Source: three-view drawing plus pictorial views. Frame: mm from the lowest corner of the part. Give positions to 0.01 mm unless a question says otherwise; leave off trailing zeros. Order: outer loops, then holes, each group sorted by start corner. A loop starts at its lowest first (then second) coordinate and runs counter-clockwise, first axis right, second up. Notation, with made-up numbers: (-5, 71) -> (10, 71) arc R15 ccw to (10, 80) -> close; hole circle Ø5 at (68.5, 26). An arc over 180 degrees is marked (long way). Answer in a Markdown table with one row per item. Add a question column.
Q1. Cut plane A-A on z = 7.53. Return the cut outline in (x, y), and give its area (3 significant figures).
Q2. Line query: line 1 along X through (y, z) = (20.5, 7). Output: solid intervals per line, ascending. Write a range as from..to.
Q3. Cut plane C-C on z = 10. Return the cut outline in (x, y).
Q4. Contact query for a flat-ended pin moving along its axis: P1, Ø6, axis at y = 8.5, z = 8, coming from the +X side. Output: stop coordinate, or through.
Q5. Cut plane B-B on y = 21. Return the cut outline in (x, z), and give its area (3 significant figures).
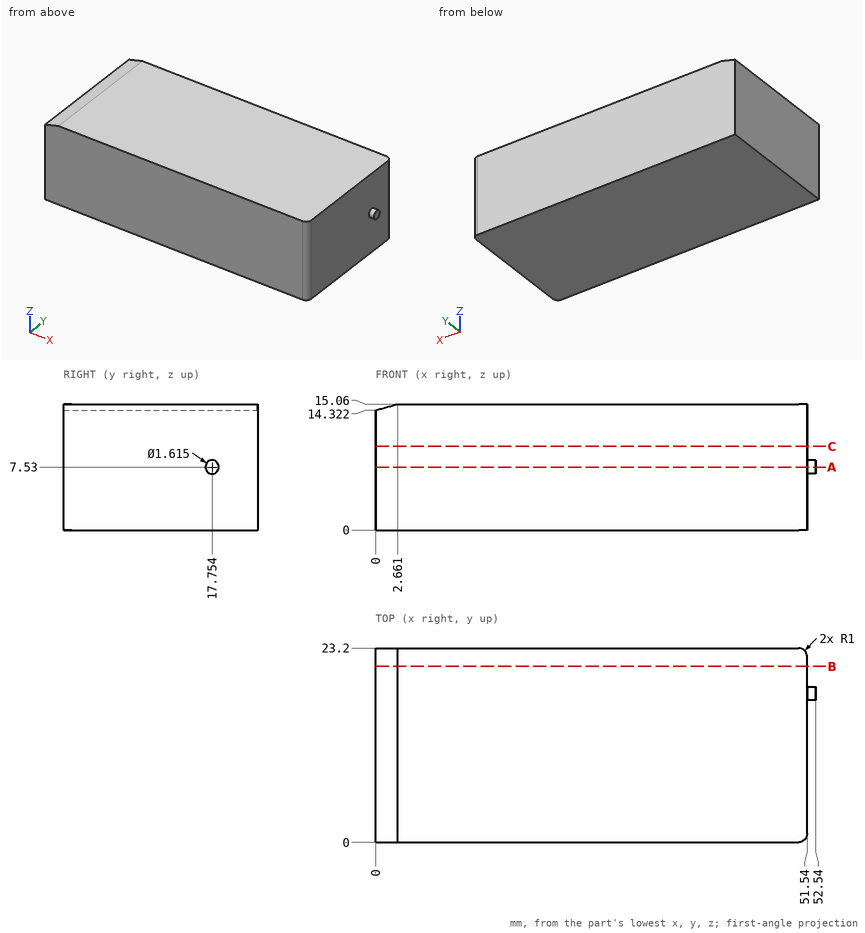
Completed:
| question | item | result |
|---|---|---|
| 1 | outline | (0, 0) -> (50.54, 0) arc R1 ccw to (51.54, 1) -> (51.54, 16.95) -> (52.54, 16.95) -> (52.54, 18.56) -> (51.54, 18.56) -> (51.54, 22.2) arc R1 ccw to (50.54, 23.2) -> (0, 23.2) -> close |
| 1 | area | 1,200 mm² |
| 2 | line 1 | x = 0..51.54 |
| 3 | outline | (0, 0) -> (50.54, 0) arc R1 ccw to (51.54, 1) -> (51.54, 22.2) arc R1 ccw to (50.54, 23.2) -> (0, 23.2) -> close |
| 4 | P1 | stops at x = 51.54 |
| 5 | outline | (0, 0) -> (51.54, 0) -> (51.54, 15.06) -> (2.66, 15.06) -> (0, 14.32) -> close |
| 5 | area | 775 mm² |
